CAD build for the part. Positions are in the model's coordinates, mm. A direction names the side the tool comes from. Give positions to 0.01 mm unless a question says otherwise; leave off trailing zeros. Loops run counter-clockwise (first coordinate to the right, second up) from the corner with the lowest first, then second, coordinate; pieces in that order, holes last. Notation, with made-up numbers: (0.5, 20.5) - (38.5, 20.5) arc R24 ccw to (38.5, 36.5) - close; hole circle Ø9 at (45, 64.5). An arc over 180 degrees is marked (long way). Return JSON: item names as keys, results as strings.
from build123d import *

# Parameters (mm, degrees)
F0_W     = 38.1
F0_H     = 38.1
F1_DEPTH = 38.1
F5_W     = 29.6418
F5_H     = 7.62
F6_DEPTH = 38.1
F8_DEPTH = 38.1


with BuildPart() as f1:
    # F0 (on Front) → F1 (new body)
    with BuildSketch(Plane.XZ):
        with Locations((19.05, 19.05)):
            Rectangle(F0_W, F0_H)
    extrude(amount=F1_DEPTH)

    # F5 (on offset) → F6 (cut)
    with BuildSketch(Plane.YZ.offset(38.1)):
        with Locations((-14.8209, 26.67)):
            Rectangle(F5_W, F5_H)
        Polygon((-8.519419, 15.24), (-38.160126, 15.24), (-38.493167, 7.62), (-8.519419, 7.62), align=None)
    extrude(amount=-F6_DEPTH, mode=Mode.SUBTRACT)

    # F7 (on offset) → F8 (cut)
    with BuildSketch(Plane.XZ.offset(38.1)):
        Polygon((38.1, 7.62), (38.1, 30.48), (12.7, 30.48), (12.7, 22.86), (28.575, 22.86), (28.575, 15.24), (12.7, 15.24), (12.7, 7.62), align=None)
    extrude(amount=-F8_DEPTH, mode=Mode.SUBTRACT)


solid = f1.part
1. Pull direction Z, two halves, no side cores. Call faces 1 (the face through (19, -19, 38.1)), 2 (the face through (14, -19, 22.86)), 3 (the face through (19, -19, 0)), 4 (the face through (15, -38.1, 32)): +Z half, -Z half, draft (parallel to the pull), parting line (faces both ways), or undercut.
Values follow:
{"face 1": "+Z half", "face 2": "undercut", "face 3": "-Z half", "face 4": "draft"}
2. Drill centre lines: probe 1 along Z at (x, y) = (8, -25); probe 2 along Z at (x, y) = (9, -3.5); probe 3 along Z at (x, y) = (31.5, -8.5). Where is each one in solid material? Low to high.
Values follow:
{"probe 1": "z = 0 to 7.62, 15.24 to 22.86, 30.48 to 38.1", "probe 2": "z = 0 to 22.86, 30.48 to 38.1", "probe 3": "z = 0 to 7.62, 30.48 to 38.1"}
3. Cut at D-D, the plane x = 32. Write the cut outline in (y, z).
Values follow:
{"outline": "(-38.1, 0) - (0, 0) - (0, 7.62) - (-38.1, 7.62) - close; (-38.1, 30.48) - (0, 30.48) - (0, 38.1) - (-38.1, 38.1) - close"}
4. Which spindle directions (+Z, -Z, +X, -X, +Y, -Y) get a long thin tool onto all of the face, cutting with end or side? Do faces 5 (the face through (12.7, -34, 27)), 6 (the face through (19, -19, 30.48)), 7 (the face through (6, -29.642, 27)), 8 (the face through (14, -19, 15.24)). Say none if no direction does.
Values follow:
{"face 5": "+X, +Y, -Y", "face 6": "+X, +Y", "face 7": "+X, -X, +Y", "face 8": "+X, -Y"}
5. Cut at C-C, the plane y = -5.5. Write the cut outline in (x, z) (3 decimals).
Values follow:
{"outline": "(0, 0) - (38.1, 0) - (38.1, 7.62) - (12.7, 7.62) - (12.7, 15.24) - (28.575, 15.24) - (28.575, 22.86) - (0, 22.86) - close; (0, 30.48) - (38.1, 30.48) - (38.1, 38.1) - (0, 38.1) - close"}
6. Cut at A-A, the plane x = 17. Write the cut outline in (y, z).
Values follow:
{"outline": "(-38.1, 0) - (0, 0) - (0, 7.62) - (-38.1, 7.62) - close; (-38.1, 15.24) - (0, 15.24) - (0, 22.86) - (-38.1, 22.86) - close; (-38.1, 30.48) - (0, 30.48) - (0, 38.1) - (-38.1, 38.1) - close"}
7. Drop flat-ended pins along their axis: P1, Ø6, axis at y = -5, z = 11.5, coming from the +X side; P2, Ø6, axis at y = -19, z = 21, coming from the +X side (3 decimals); P3, Ø2.5, axis at x = 6.5, z = 25, coming from the +Y side. Give the stop position or say it passes through.
Values follow:
{"P1": "stops at x = 12.7", "P2": "stops at x = 28.575", "P3": "stops at y = -29.64"}
8. Cut at B-B, the plane y = -15.5. Write the cut outline in (x, z) (3 decimals).
Values follow:
{"outline": "(0, 0) - (38.1, 0) - (38.1, 7.62) - (0, 7.62) - close; (0, 15.24) - (28.575, 15.24) - (28.575, 22.86) - (0, 22.86) - close; (0, 30.48) - (38.1, 30.48) - (38.1, 38.1) - (0, 38.1) - close"}
